from build123d import *

# Parameters (mm, degrees)
SKETCH1_W                       = 50.8
SKETCH1_H                       = 50.8
BOSS_EXTRUDE1_DEPTH             = 2.54
HOLES_FOR_ARMS_D                = 3.4
HOLES_FOR_STRUCTURE_D           = 3.4
CORNERS_START                   = -2.54
CORNERS_DEPTH                   = 39.550715072
MIRROR_START                    = -2.54
MIRROR_OF_CORNER_2_COPY_1_DEPTH = 39.550715072
SKETCH16_W                      = 2.54
SKETCH16_H                      = 2.54
CUT_EXTRUDE1_DEPTH              = 2.54
SKETCH17_R                      = 1.905
BOSS_EXTRUDE4_DEPTH             = 2.54
SKETCH17_6_R                    = 1.905
CUT_EXTRUDE2_DEPTH              = 37.010715072
SKETCH18_R                      = 0.9906
CUT_EXTRUDE3_DEPTH              = 2.54
SKETCH19_W                      = 2.54
SKETCH19_H                      = 15.24
CUT_EXTRUDE4_DEPTH              = 37.010715072


with BuildPart() as part:
    # Sketch1 → Boss-Extrude1 (new body)
    with BuildSketch(Plane(origin=(0, 0, 0), x_dir=(1, 0, 0), z_dir=(0, 1, 0))):
        Rectangle(SKETCH1_W, SKETCH1_H)
    extrude(amount=BOSS_EXTRUDE1_DEPTH)

    # holes for arms (through all)
    with Locations(Plane(origin=(0, 2.54, 0), x_dir=(1, 0, 0), z_dir=(0, 1, 0))):
        with Locations((-20.32, -11.684), (-20.32, 11.684)):
            Hole(HOLES_FOR_ARMS_D / 2)

    # holes for structure (through all)
    with Locations(Plane(origin=(0, 2.54, 0), x_dir=(1, 0, 0), z_dir=(0, 1, 0))):
        with Locations((17.78, -17.78), (17.78, 17.78)):
            Hole(HOLES_FOR_STRUCTURE_D / 2)

    # Sketch12 → corners (cut)
    with BuildSketch(Plane(origin=(0, 2.54, 0), x_dir=(1, 0, 0), z_dir=(0, 1, 0)).offset(CORNERS_START)):
        Polygon((-25.4, -25.4), (-20.909871939, -25.4), (-25.4, -20.909871939), align=None)
    corners = extrude(amount=CORNERS_DEPTH, mode=Mode.SUBTRACT)

    # mirror of corner: corners across plane
    add(corners.mirror(Plane.ZY), mode=Mode.SUBTRACT)

    # mirror of corner 2: corners across plane
    add(corners.mirror(Plane(origin=(0, 0, 0), x_dir=(1, 0, 0), z_dir=(0, 0, -1))), mode=Mode.SUBTRACT)

    # mirror of corner 2 copy 1 sketch → mirror of corner 2 copy 1 (cut)
    with BuildSketch(Plane(origin=(0, 2.54, 0), x_dir=(-1, 0, 0), z_dir=(0, 1, 0)).offset(MIRROR_START)):
        Polygon((-25.4, -25.4), (-20.909871939, -25.4), (-25.4, -20.909871939), align=None)
    extrude(amount=MIRROR_OF_CORNER_2_COPY_1_DEPTH, mode=Mode.SUBTRACT)

    # Sketch16 → Cut-Extrude1 (cut)
    with BuildSketch(Plane(origin=(0, 2.54, 0), x_dir=(1, 0, 0), z_dir=(0, 1, 0))):
        with Locations((22.86, -8.89)):
            Rectangle(SKETCH16_W, SKETCH16_H)
        with Locations((22.86, 8.89)):
            Rectangle(SKETCH16_W, SKETCH16_H)
    extrude(amount=-CUT_EXTRUDE1_DEPTH, mode=Mode.SUBTRACT)

    # Sketch17 → Boss-Extrude4 (add, through all)
    with BuildSketch(Plane(origin=(0, 2.54, 0), x_dir=(1, 0, 0), z_dir=(0, 1, 0))):
        with Locations((-2.794, 11.684)):
            Circle(SKETCH17_R)
    extrude(amount=-BOSS_EXTRUDE4_DEPTH)

    # Sketch17<6> → Cut-Extrude2 (cut, through all)
    with BuildSketch(Plane(origin=(0, 2.54, 0), x_dir=(1, 0, 0), z_dir=(0, 1, 0))):
        with Locations(Location((-2.794, 11.684, 0), (0, 0, 270))):
            Circle(SKETCH17_6_R)
    extrude(amount=-CUT_EXTRUDE2_DEPTH, mode=Mode.SUBTRACT)

    # Sketch18 → Cut-Extrude3 (cut)
    with BuildSketch(Plane(origin=(0, 2.54, 0), x_dir=(1, 0, 0), z_dir=(0, 1, 0))):
        with Locations(Location((-2.794, 19.05, 0), (0, 0, 270))):
            Circle(SKETCH18_R)
        with Locations(Location((-2.794, -9.3472, 0), (0, 0, 270))):
            Circle(SKETCH18_R)
        with BuildLine():
            Line((-5.294, 5.846834592), (-5.294, -0.153165408))
            Line((-5.294, -0.153165408), (-0.294, -0.153165408))
            Line((-0.294, -0.153165408), (-0.294, 5.846834592))
            ThreePointArc((-0.294, 5.846834592), (-2.794, 18.034), (-5.294, 5.846834592))
        make_face()
    extrude(amount=-CUT_EXTRUDE3_DEPTH, mode=Mode.SUBTRACT)

    # Sketch19 → Cut-Extrude4 (cut, through all)
    with BuildSketch(Plane(origin=(0, 2.54, 0), x_dir=(1, 0, 0), z_dir=(0, 1, 0))):
        with Locations((22.86, 0)):
            Rectangle(SKETCH19_W, SKETCH19_H)
    extrude(amount=-CUT_EXTRUDE4_DEPTH, mode=Mode.SUBTRACT)


solid = part.part
Can you work these out from the model? Positions are in its coordinate system, mm. A direction names the side the tool comes from. Coordinates: 2 decimals unless noted, no trailing zeros. Write each loop counter-clockwise with the first axis right and the second up, starting at its lowest first coordinate (ties: lowest second). Pieces come first, ordered by that corner, then holes. Notation, with made-up numbers: (73, -37) -> (90, -37) arc R20 ccw to (90, -33) -> close; hole circle Ø4 at (-3, 44). An arc over 180 degrees is marked (long way). Write each question's results on one line, items separated by ' | '. Start each with the question number.
Item 1: If we section it at A-A, the plane z = 17.78: Write out the boundary of the cut face in (x, y).
Item 2: Please list where these lines run through material, in increasing order: probe 1 along X at (y, z) = (2.05, -2); probe 2 along Z at (x, y) = (-20.32, 1.1); probe 3 along X at (y, z) = (0.6, 5.5).
Item 3: If we section it at C-C, the plane y = 1.95: Count the separate pieces of the cut face and the enclosed holes in it, and give its area (3 significant figures).
Item 4: If we section it at B-B, the plane x = -20.32: Write out the boundary of the cut face in (y, z), and give its area (3 significant figures).
Item 5: On a 3-axis mill with a long thin cutter (end or side, diameter ignored), from which of +Z, -Z, +X, -X, +Y, -Y can I reach the whole of each face in a straight line? I mean faces 5 (the flat face through (23, 1, -10.16)), 6 (the flat face through (25.4, 1, 0)). Say none if no direction works.
Item 6: Thinking about a two-plate mould opening in Z: for faces 1 (the cylindrical face through (-3.173, 1.288, 10.262)), 2 (the flat face through (0, 1, -25.4)), 3 (the cylindrical face through (16.21, 1.25, -17.13)), 4 (the flat face through (-25.4, 1, 0)), which applies, released by +Z, released by -Z, zero draft, split by the parting line, or undercut?
Item 7: I'm going to push flat-ended pins straight in: P1, Ø1.3, axis at x = 22.5, y = 1, coming from the +Z side; P2, Ø11.5, axis at x = -2.794, z = -11.684, coming from the -Y side; P3, Ø0.8, axis at x = 22.5, y = 1, coming from the -Z side. Where does each tip first touch, or does it pass through?
Item 8: If we section it at D-D, the plane x = 2: Write out the boundary of the cut face in (y, z).
Answer block:
1) outline: (-25.4, 0) -> (16.08, 0) -> (16.08, 2.54) -> (-25.4, 2.54) -> close; (19.48, 0) -> (25.4, 0) -> (25.4, 2.54) -> (19.48, 2.54) -> close
2) probe 1: -25.4 to -5.29, -0.29 to 21.59, 24.13 to 25.4 | probe 2: -25.4 to -13.38, -9.98 to 9.98, 13.38 to 25.4 | probe 3: -25.4 to 21.59, 24.13 to 25.4
3) separate pieces: 1 | enclosed holes: 8 | area: 2,290 mm²
4) outline: (0, -25.4) -> (2.54, -25.4) -> (2.54, -13.38) -> (0, -13.38) -> close; (0, -9.98) -> (2.54, -9.98) -> (2.54, 9.98) -> (0, 9.98) -> close; (0, 13.38) -> (2.54, 13.38) -> (2.54, 25.4) -> (0, 25.4) -> close | area: 112 mm²
5) face 5: +Y, -Y | face 6: +Z, -Z, +X, +Y, -Y
6) face 1: undercut | face 2: released by -Z | face 3: undercut | face 4: zero draft
7) P1: z = 24.46 | P2: through | P3: z = -24.21
8) outline: (0, -25.4) -> (2.54, -25.4) -> (2.54, -15.85) -> (0, -15.85) -> close; (0, -7.52) -> (2.54, -7.52) -> (2.54, 25.4) -> (0, 25.4) -> close
